```python
from build123d import *

# Parameters (mm, degrees)
F0_R     = 65
F1_DEPTH = 69
F2_DEPTH = 7
F3_R     = 65
F4_DEPTH = 7


with BuildPart() as f1:
    # F0 (on Top) → F1 (new body)
    with BuildSketch(Plane.XY):
        with BuildLine():
            Line((-5.939693756, -76.2), (5.939693756, -76.2))
            ThreePointArc((5.939693756, -76.2), (54.0449810894, -54.0449810894), (76.2, -5.939693756))
            Line((76.2, -5.939693756), (76.2, 5.939693756))
            ThreePointArc((76.2, 5.939693756), (54.0449810894, 54.0449810894), (5.939693756, 76.2))
            Line((5.939693756, 76.2), (-5.939693756, 76.2))
            ThreePointArc((-5.939693756, 76.2), (-54.0449810894, 54.0449810894), (-76.2, 5.939693756))
            Line((-76.2, 5.939693756), (-76.2, -5.939693756))
            ThreePointArc((-76.2, -5.939693756), (-54.0449810894, -54.0449810894), (-5.939693756, -76.2))
        make_face()
        Circle(F0_R, mode=Mode.SUBTRACT)
    extrude(amount=F1_DEPTH)

    # F0 (on Top) → F2 (join)
    with BuildSketch(Plane.XY):
        with BuildLine():
            Line((5.939693756, -76.2), (76.2, -76.2))
            Line((76.2, -76.2), (76.2, -5.939693756))
            ThreePointArc((76.2, -5.939693756), (54.0449810894, -54.0449810894), (5.939693756, -76.2))
        make_face()
        with BuildLine():
            ThreePointArc((-5.939693756, -76.2), (0, -76.4311452349), (5.939693756, -76.2))
            Line((5.939693756, -76.2), (-5.939693756, -76.2))
        make_face()
        with BuildLine():
            Line((-5.939693756, -76.2), (5.939693756, -76.2))
            ThreePointArc((5.939693756, -76.2), (54.0449810894, -54.0449810894), (76.2, -5.939693756))
            Line((76.2, -5.939693756), (76.2, 5.939693756))
            ThreePointArc((76.2, 5.939693756), (54.0449810894, 54.0449810894), (5.939693756, 76.2))
            Line((5.939693756, 76.2), (-5.939693756, 76.2))
            ThreePointArc((-5.939693756, 76.2), (-54.0449810894, 54.0449810894), (-76.2, 5.939693756))
            Line((-76.2, 5.939693756), (-76.2, -5.939693756))
            ThreePointArc((-76.2, -5.939693756), (-54.0449810894, -54.0449810894), (-5.939693756, -76.2))
        make_face()
        Circle(F0_R, mode=Mode.SUBTRACT)
        with BuildLine():
            Line((76.2, 5.939693756), (76.2, -5.939693756))
            ThreePointArc((76.2, -5.939693756), (76.3733370648, -2.9720948014), (76.4311452349, 0))
            ThreePointArc((76.4311452349, 0), (76.3733370648, 2.9720948014), (76.2, 5.939693756))
        make_face()
        with BuildLine():
            Line((-76.2, -76.2), (-5.939693756, -76.2))
            ThreePointArc((-5.939693756, -76.2), (-54.0449810894, -54.0449810894), (-76.2, -5.939693756))
            Line((-76.2, -5.939693756), (-76.2, -76.2))
        make_face()
        with BuildLine():
            ThreePointArc((5.939693756, 76.2), (54.0449810894, 54.0449810894), (76.2, 5.939693756))
            Line((76.2, 5.939693756), (76.2, 76.2))
            Line((76.2, 76.2), (5.939693756, 76.2))
        make_face()
        with BuildLine():
            ThreePointArc((-76.2, 5.939693756), (-76.4311452349, 0), (-76.2, -5.939693756))
            Line((-76.2, -5.939693756), (-76.2, 5.939693756))
        make_face()
        with BuildLine():
            Line((-5.939693756, 76.2), (5.939693756, 76.2))
            ThreePointArc((5.939693756, 76.2), (0, 76.4311452349), (-5.939693756, 76.2))
        make_face()
        with BuildLine():
            Line((-76.2, 76.2), (-76.2, 5.939693756))
            ThreePointArc((-76.2, 5.939693756), (-54.0449810894, 54.0449810894), (-5.939693756, 76.2))
            Line((-5.939693756, 76.2), (-76.2, 76.2))
        make_face()
    extrude(amount=-F2_DEPTH)

    # F3 (on face) → F4 (join)
    with BuildSketch(Plane.XY.offset(69)):
        with BuildLine():
            Line((5.939693756, -76.2), (76.2, -76.2))
            Line((76.2, -76.2), (76.2, -5.939693756))
            ThreePointArc((76.2, -5.939693756), (54.0449810894, -54.0449810894), (5.939693756, -76.2))
        make_face()
        with BuildLine():
            ThreePointArc((-5.939693756, -76.2), (0, -76.4311452349), (5.939693756, -76.2))
            Line((5.939693756, -76.2), (-5.939693756, -76.2))
        make_face()
        with BuildLine():
            Line((-5.939693756, -76.2), (5.939693756, -76.2))
            ThreePointArc((5.939693756, -76.2), (54.0449810894, -54.0449810894), (76.2, -5.939693756))
            Line((76.2, -5.939693756), (76.2, 5.939693756))
            ThreePointArc((76.2, 5.939693756), (54.0449810894, 54.0449810894), (5.939693756, 76.2))
            Line((5.939693756, 76.2), (-5.939693756, 76.2))
            ThreePointArc((-5.939693756, 76.2), (-54.0449810894, 54.0449810894), (-76.2, 5.939693756))
            Line((-76.2, 5.939693756), (-76.2, -5.939693756))
            ThreePointArc((-76.2, -5.939693756), (-54.0449810894, -54.0449810894), (-5.939693756, -76.2))
        make_face()
        Circle(F3_R, mode=Mode.SUBTRACT)
        with BuildLine():
            Line((76.2, 5.939693756), (76.2, -5.939693756))
            ThreePointArc((76.2, -5.939693756), (76.3733370648, -2.9720948014), (76.4311452349, 0))
            ThreePointArc((76.4311452349, 0), (76.3733370648, 2.9720948014), (76.2, 5.939693756))
        make_face()
        with BuildLine():
            Line((-76.2, -76.2), (-5.939693756, -76.2))
            ThreePointArc((-5.939693756, -76.2), (-54.0449810894, -54.0449810894), (-76.2, -5.939693756))
            Line((-76.2, -5.939693756), (-76.2, -76.2))
        make_face()
        with BuildLine():
            ThreePointArc((5.939693756, 76.2), (54.0449810894, 54.0449810894), (76.2, 5.939693756))
            Line((76.2, 5.939693756), (76.2, 76.2))
            Line((76.2, 76.2), (5.939693756, 76.2))
        make_face()
        with BuildLine():
            ThreePointArc((-76.2, 5.939693756), (-76.4311452349, 0), (-76.2, -5.939693756))
            Line((-76.2, -5.939693756), (-76.2, 5.939693756))
        make_face()
        with BuildLine():
            Line((-5.939693756, 76.2), (5.939693756, 76.2))
            ThreePointArc((5.939693756, 76.2), (0, 76.4311452349), (-5.939693756, 76.2))
        make_face()
        with BuildLine():
            Line((-76.2, 76.2), (-76.2, 5.939693756))
            ThreePointArc((-76.2, 5.939693756), (-54.0449810894, 54.0449810894), (-5.939693756, 76.2))
            Line((-5.939693756, 76.2), (-76.2, 76.2))
        make_face()
    extrude(amount=F4_DEPTH)


solid = f1.part
```
Model file for the job. Use its own axes, mm. A direction names the side the tool comes from. Coordinates: 2 decimals unless noted, no trailing zeros. Loops run counter-clockwise (first coordinate to the right, second up) from the corner with the lowest first, then second, coordinate; pieces in that order, holes last. Notation, with made-up numbers: M 25,69 L 45,69 A20 cw 45,103 Z; hole C -7.75,-21 d5. An arc over 180 degrees is marked long. Use CSV: the item, a comma, the result in double quotes. Start each with the question number.
1. Band-saw the part on B-B, the plane x = 0. List the corners of the cut face in (y, z), then the cut area to 3 significant figures.
2. Tool access for faces 4 (the flat face through (-76.2, 42, 72)), 5 (the flat face through (-76.2, 0, 34)), 6 (the flat face through (-76.2, -41, 72)), 7 (the flat face through (76.2, 41, 72)), 8 (the flat face through (76.2, -42, -3)): list every direction of +Z, -Z, +X, -X, +Y, -Y with a clear straight run to the whole face (end or side of a thin tool).
3. Flat gauge pins, fed straight in: pin 1 (3.5 mm diameter, centred on y = 52.5, z = -2.5, fed in from -X); pin 2 (10 mm diameter, centred on x = -33, z = 44.5, fed in from +Y); pin 3 (3.5 mm diameter, centred on x = -52.5, z = 71, fed in from -Y); pin 4 (3 mm diameter, centred on x = -51, y = 36.5, fed in from -Z). Where does each tip first touch, or does it go through?
4. Band-saw the part on A-A, the plane y = 2. List the corners of the cut face in (x, z), then the cut area to 3 significant figures.
5. Band-saw the part on C-C, the plane z = 58.5. List the corners of the cut face in (x, y), then the cut area to 3 significant figures.
6. Probe probe 1 along Y at (x, z) = (0, 41); probe 2 along Y at (x, z) = (19, 7.5); probe 3 along X at (y, z) = (51, 8.5). List the from-to ranges inside material, lowest first. Write a range as [from, to].
7. Two-plate mould, pull along Z, no slides. Class faces 1 (the flat face through (-59, -62, 69)), 2 (the flat face through (-76.2, 42, -3)), 3 (the flat face through (-69, 1, -7)): pulls with the +Z half, pulls with the -Z half, needs draft (parallel to the pull), parting line crosses it, or undercut.
Entries:
1,outline,"M -76.43,-7 L -65,-7 L -65,76 L -76.43,76 L -76.43,69 L -76.2,69 L -76.2,0 L -76.43,0 Z; M 65,-7 L 76.43,-7 L 76.43,0 L 76.2,0 L 76.2,69 L 76.43,69 L 76.43,76 L 65,76 Z"
1,area,"1,870 mm2"
2,face 4,"+Z, -Z, -X, +Y"
2,face 5,"-X, +Y, -Y"
2,face 6,"+Z, -Z, -X, -Y"
2,face 7,"+Z, -Z, +X, +Y"
2,face 8,"+Z, -Z, +X, -Y"
3,pin 1,"stops at x = -76.2"
3,pin 2,"stops at y = 71.12"
3,pin 3,"stops at y = -76.2"
3,pin 4,"passes through"
4,outline,"M -76.4,-7 L -64.97,-7 L -64.97,76 L -76.4,76 L -76.4,69 L -76.2,69 L -76.2,0 L -76.4,0 Z; M 64.97,-7 L 76.4,-7 L 76.4,0 L 76.2,0 L 76.2,69 L 76.4,69 L 76.4,76 L 64.97,76 Z"
4,area,"1,870 mm2"
5,outline,"M -76.2,-5.94 A76.43 ccw -5.94,-76.2 L 5.94,-76.2 A76.43 ccw 76.2,-5.94 L 76.2,5.94 A76.43 ccw 5.94,76.2 L -5.94,76.2 A76.43 ccw -76.2,5.94 Z; hole C 0,0 d130"
5,area,"5,070 mm2"
6,probe 1,"y = [-76.2, -65], [65, 76.2]"
6,probe 2,"y = [-74.03, -62.16], [62.16, 74.03]"
6,probe 3,"x = [-56.93, -40.3], [40.3, 56.93]"
7,face 1,"undercut"
7,face 2,"needs draft"
7,face 3,"pulls with the -Z half"
